Geometry check sheet. Reference: the model listing, model coordinates, mm. A direction names the side the tool comes from. Round coordinates to 2 decimals unless told otherwise and drop trailing zeros. Write each loop counter-clockwise with the first axis right and the second up, starting at its lowest first coordinate (ties: lowest second). Pieces come first, ordered by that corner, then holes. Notation, with made-up numbers: (66, 88) - (88, 88) arc R23 cw to (88, 117) - close; hole circle Ø5 at (-22, 34.5). An arc over 180 degrees is marked (long way). Return JSON: item names as keys, results as strings.
```python
from build123d import *

# Parameters (mm, degrees)
CROQUIS1_R              = 3.1
SALIENTE_EXTRUIR1_DEPTH = 12


with BuildPart() as part:
    # Croquis1 → Saliente-Extruir1 (new body)
    with BuildSketch(Plane.XY):
        Polygon((331.272984938, 614.597621835), (321.632458304, 1225.948656715), (1286.013878227, 1225.948656715), (1286.013878227, 614.597621835), align=None)
        with Locations((1170.33582343, 889.102037351)):
            Circle(CROQUIS1_R, mode=Mode.SUBTRACT)
        with Locations((1220.33582343, 889.102037351)):
            Circle(CROQUIS1_R, mode=Mode.SUBTRACT)
        with Locations((1220.33582343, 953.102037351)):
            Circle(CROQUIS1_R, mode=Mode.SUBTRACT)
        with Locations((1170.33582343, 953.102037351)):
            Circle(CROQUIS1_R, mode=Mode.SUBTRACT)
        with Locations((435.286525189, 859.802037351)):
            Circle(CROQUIS1_R, mode=Mode.SUBTRACT)
        with Locations((370.33582343, 923.276635067)):
            Circle(CROQUIS1_R, mode=Mode.SUBTRACT)
        with Locations((435.286525189, 982.402037351)):
            Circle(CROQUIS1_R, mode=Mode.SUBTRACT)
        with Locations((492.93582343, 923.276635067)):
            Circle(CROQUIS1_R, mode=Mode.SUBTRACT)
        with BuildLine():
            Line((394.578464117, 962.402037351), (468.693182742, 962.402037351))
            ThreePointArc((468.693182742, 962.402037351), (472.93582343, 962.402037351), (472.93582343, 958.159396664))
            Line((472.93582343, 958.159396664), (472.93582343, 884.044678039))
            ThreePointArc((472.93582343, 884.044678039), (472.93582343, 879.802037351), (468.693182742, 879.802037351))
            Line((468.693182742, 879.802037351), (394.578464117, 879.802037351))
            ThreePointArc((394.578464117, 879.802037351), (390.33582343, 879.802037351), (390.33582343, 884.044678039))
            Line((390.33582343, 884.044678039), (390.33582343, 958.159396664))
            ThreePointArc((390.33582343, 958.159396664), (390.33582343, 962.402037351), (394.578464117, 962.402037351))
        make_face(mode=Mode.SUBTRACT)
        with BuildLine():
            Line((742.33582343, 1208.859396664), (742.33582343, 1193.344678039))
            ThreePointArc((742.33582343, 1193.344678039), (742.33582343, 1189.102037351), (738.093182742, 1189.102037351))
            Line((738.093182742, 1189.102037351), (690.578464117, 1189.102037351))
            ThreePointArc((690.578464117, 1189.102037351), (686.33582343, 1189.102037351), (686.33582343, 1193.344678039))
            Line((686.33582343, 1193.344678039), (686.33582343, 1208.859396664))
            ThreePointArc((686.33582343, 1208.859396664), (686.33582343, 1213.102037351), (690.578464117, 1213.102037351))
            Line((690.578464117, 1213.102037351), (738.093182742, 1213.102037351))
            ThreePointArc((738.093182742, 1213.102037351), (742.33582343, 1213.102037351), (742.33582343, 1208.859396664))
        make_face(mode=Mode.SUBTRACT)
        with BuildLine():
            Line((934.33582343, 648.859396664), (934.33582343, 633.344678039))
            ThreePointArc((934.33582343, 633.344678039), (934.33582343, 629.102037351), (930.093182742, 629.102037351))
            Line((930.093182742, 629.102037351), (882.578464117, 629.102037351))
            ThreePointArc((882.578464117, 629.102037351), (878.33582343, 629.102037351), (878.33582343, 633.344678039))
            Line((878.33582343, 633.344678039), (878.33582343, 648.859396664))
            ThreePointArc((878.33582343, 648.859396664), (878.33582343, 653.102037351), (882.578464117, 653.102037351))
            Line((882.578464117, 653.102037351), (930.093182742, 653.102037351))
            ThreePointArc((930.093182742, 653.102037351), (934.33582343, 653.102037351), (934.33582343, 648.859396664))
        make_face(mode=Mode.SUBTRACT)
        with BuildLine():
            Line((690.578464117, 653.102037351), (738.093182742, 653.102037351))
            ThreePointArc((738.093182742, 653.102037351), (742.33582343, 653.102037351), (742.33582343, 648.859396664))
            Line((742.33582343, 648.859396664), (742.33582343, 633.344678039))
            ThreePointArc((742.33582343, 633.344678039), (742.33582343, 629.102037351), (738.093182742, 629.102037351))
            Line((738.093182742, 629.102037351), (690.578464117, 629.102037351))
            ThreePointArc((690.578464117, 629.102037351), (686.33582343, 629.102037351), (686.33582343, 633.344678039))
            Line((686.33582343, 633.344678039), (686.33582343, 648.859396664))
            ThreePointArc((686.33582343, 648.859396664), (686.33582343, 653.102037351), (690.578464117, 653.102037351))
        make_face(mode=Mode.SUBTRACT)
        with BuildLine():
            Line((1220.33582343, 671.102037351), (400.33582343, 671.102037351))
            ThreePointArc((400.33582343, 671.102037351), (393.264755618, 674.03096954), (390.33582343, 681.102037351))
            Line((390.33582343, 681.102037351), (390.33582343, 757.264835053))
            ThreePointArc((390.33582343, 757.264835053), (390.808048943, 760.301529527), (392.180126095, 763.05142308))
            Line((392.180126095, 763.05142308), (443.646345243, 835.588625378))
            ThreePointArc((443.646345243, 835.588625378), (447.212155883, 838.686458556), (451.802042577, 839.802037351))
            Line((451.802042577, 839.802037351), (502.93582343, 839.802037351))
            ThreePointArc((502.93582343, 839.802037351), (510.006891241, 842.73096954), (512.93582343, 849.802037351))
            Line((512.93582343, 849.802037351), (512.93582343, 992.402037351))
            ThreePointArc((512.93582343, 992.402037351), (510.006891241, 999.473105163), (502.93582343, 1002.402037351))
            Line((502.93582343, 1002.402037351), (451.802042577, 1002.402037351))
            ThreePointArc((451.802042577, 1002.402037351), (447.212155883, 1003.517616147), (443.646345243, 1006.615449325))
            Line((443.646345243, 1006.615449325), (392.180126095, 1079.152651623))
            ThreePointArc((392.180126095, 1079.152651623), (390.808048943, 1081.902545176), (390.33582343, 1084.93923965))
            Line((390.33582343, 1084.93923965), (390.33582343, 1161.102037351))
            ThreePointArc((390.33582343, 1161.102037351), (393.264755618, 1168.173105163), (400.33582343, 1171.102037351))
            Line((400.33582343, 1171.102037351), (1220.33582343, 1171.102037351))
            ThreePointArc((1220.33582343, 1171.102037351), (1227.406891241, 1168.173105163), (1230.33582343, 1161.102037351))
            Line((1230.33582343, 1161.102037351), (1230.33582343, 1068.903333434))
            ThreePointArc((1230.33582343, 1068.903333434), (1230.177434198, 1067.130567942), (1229.707283932, 1065.413959843))
            Line((1229.707283932, 1065.413959843), (1197.759992837, 979.61266376))
            ThreePointArc((1197.759992837, 979.61266376), (1194.094067546, 974.889433139), (1188.388532335, 973.102037351))
            Line((1188.388532335, 973.102037351), (1160.33582343, 973.102037351))
            ThreePointArc((1160.33582343, 973.102037351), (1153.264755618, 970.173105163), (1150.33582343, 963.102037351))
            Line((1150.33582343, 963.102037351), (1150.33582343, 943.102037351))
            ThreePointArc((1150.33582343, 943.102037351), (1153.264755618, 936.03096954), (1160.33582343, 933.102037351))
            Line((1160.33582343, 933.102037351), (1220.33582343, 933.102037351))
            ThreePointArc((1220.33582343, 933.102037351), (1227.406891241, 930.173105163), (1230.33582343, 923.102037351))
            Line((1230.33582343, 923.102037351), (1230.33582343, 919.102037351))
            ThreePointArc((1230.33582343, 919.102037351), (1227.406891241, 912.03096954), (1220.33582343, 909.102037351))
            Line((1220.33582343, 909.102037351), (1160.33582343, 909.102037351))
            ThreePointArc((1160.33582343, 909.102037351), (1153.264755618, 906.173105163), (1150.33582343, 899.102037351))
            Line((1150.33582343, 899.102037351), (1150.33582343, 879.102037351))
            ThreePointArc((1150.33582343, 879.102037351), (1153.264755618, 872.03096954), (1160.33582343, 869.102037351))
            Line((1160.33582343, 869.102037351), (1188.388532335, 869.102037351))
            ThreePointArc((1188.388532335, 869.102037351), (1194.094067546, 867.314641564), (1197.759992837, 862.591410943))
            Line((1197.759992837, 862.591410943), (1229.707283932, 776.79011486))
            ThreePointArc((1229.707283932, 776.79011486), (1230.177434198, 775.073506761), (1230.33582343, 773.300741269))
            Line((1230.33582343, 773.300741269), (1230.33582343, 681.102037351))
            ThreePointArc((1230.33582343, 681.102037351), (1227.406891241, 674.03096954), (1220.33582343, 671.102037351))
        make_face(mode=Mode.SUBTRACT)
        with BuildLine():
            Line((786.578464117, 653.102037351), (834.093182742, 653.102037351))
            ThreePointArc((834.093182742, 653.102037351), (838.33582343, 653.102037351), (838.33582343, 648.859396664))
            Line((838.33582343, 648.859396664), (838.33582343, 635.344678039))
            ThreePointArc((838.33582343, 635.344678039), (838.33582343, 631.102037351), (834.093182742, 631.102037351))
            Line((834.093182742, 631.102037351), (786.578464117, 631.102037351))
            ThreePointArc((786.578464117, 631.102037351), (782.33582343, 631.102037351), (782.33582343, 635.344678039))
            Line((782.33582343, 635.344678039), (782.33582343, 648.859396664))
            ThreePointArc((782.33582343, 648.859396664), (782.33582343, 653.102037351), (786.578464117, 653.102037351))
        make_face(mode=Mode.SUBTRACT)
        with BuildLine():
            Line((934.33582343, 1208.859396664), (934.33582343, 1193.344678039))
            ThreePointArc((934.33582343, 1193.344678039), (934.33582343, 1189.102037351), (930.093182742, 1189.102037351))
            Line((930.093182742, 1189.102037351), (882.578464117, 1189.102037351))
            ThreePointArc((882.578464117, 1189.102037351), (878.33582343, 1189.102037351), (878.33582343, 1193.344678039))
            Line((878.33582343, 1193.344678039), (878.33582343, 1208.859396664))
            ThreePointArc((878.33582343, 1208.859396664), (878.33582343, 1213.102037351), (882.578464117, 1213.102037351))
            Line((882.578464117, 1213.102037351), (930.093182742, 1213.102037351))
            ThreePointArc((930.093182742, 1213.102037351), (934.33582343, 1213.102037351), (934.33582343, 1208.859396664))
        make_face(mode=Mode.SUBTRACT)
        with BuildLine():
            Line((838.33582343, 1206.859396664), (838.33582343, 1193.344678039))
            ThreePointArc((838.33582343, 1193.344678039), (838.33582343, 1189.102037351), (834.093182742, 1189.102037351))
            Line((834.093182742, 1189.102037351), (786.578464117, 1189.102037351))
            ThreePointArc((786.578464117, 1189.102037351), (782.33582343, 1189.102037351), (782.33582343, 1193.344678039))
            Line((782.33582343, 1193.344678039), (782.33582343, 1206.859396664))
            ThreePointArc((782.33582343, 1206.859396664), (782.33582343, 1211.102037351), (786.578464117, 1211.102037351))
            Line((786.578464117, 1211.102037351), (834.093182742, 1211.102037351))
            ThreePointArc((834.093182742, 1211.102037351), (838.33582343, 1211.102037351), (838.33582343, 1206.859396664))
        make_face(mode=Mode.SUBTRACT)
    extrude(amount=SALIENTE_EXTRUIR1_DEPTH)


solid = part.part
```
(1) Material ranges on line 1 along Y through (x, z) = (472, 5.5); line 2 along Y through (x, z) = (724, 5.25); line 3 along Y through (x, z) = (843, 1.5), recorded low to high. Write a range as [from, to].
Response values:
{"line 1": "y = [614.6, 671.1], [839.8, 879.17], [963.04, 1002.4], [1171.1, 1225.95]", "line 2": "y = [614.6, 629.1], [653.1, 671.1], [1171.1, 1189.1], [1213.1, 1225.95]", "line 3": "y = [614.6, 671.1], [1171.1, 1225.95]"}
(2) Section check A-A, the plane y = 722. Enter the section's corners in (x, z).
Response values:
{"outline": "(329.58, 0) - (390.34, 0) - (390.34, 12) - (329.58, 12) - close; (1230.34, 0) - (1286.01, 0) - (1286.01, 12) - (1230.34, 12) - close"}
(3) Gauge pin test, flat ends, axial feed: pin 1 (5 mm diameter, centred on x = 1170.34, y = 889.1, fed in from +Z); pin 2 (2 mm diameter, centred on y = 921, z = 6, fed in from -X); pin 3 (6 mm diameter, centred on y = 1111, z = 3, fed in from -X); pin 4 (3 mm diameter, centred on y = 692.5, z = 7, fed in from -X). Record the tip position at first contact, or that the pin passes through.
Response values:
{"pin 1": "passes through", "pin 2": "stops at x = 326.43", "pin 3": "stops at x = 323.4", "pin 4": "stops at x = 330.02"}
(4) Release check for a two-part mould opening along Y. For faces 3 (the face through (1213.51, 820.29, 5.92)), 4 (the face through (842, 1193, 12)) record: pulls with the +Y half, pulls with the -Y half, needs draft (parallel to the pull), parting line crosses it, or undercut.
Response values:
{"face 3": "undercut", "face 4": "needs draft"}
(5) Section check B-B, the plane x = 628.5. Enter the section's corners in (y, z).
Response values:
{"outline": "(614.6, 0) - (671.1, 0) - (671.1, 12) - (614.6, 12) - close; (1171.1, 0) - (1225.95, 0) - (1225.95, 12) - (1171.1, 12) - close"}
(6) Access from +Z, -Z, +X, -X, +Y, -Y to the whole of each face (thin tool, end or side, straight path). Record for faces 1 (the face through (1213.957, 1023.114, 5.916)), 2 (the face through (842, 1193, 0)).
Response values:
{"face 1": "+Z, -Z", "face 2": "-Z, +X, -X, +Y, -Y"}
(7) Section check C-C, the plane z = 2.5. Give the number of separate pieces and of enclosed holes in the cut face, plus the area to 3 significant figures.
Response values:
{"separate pieces": "1", "enclosed holes": "16", "area": "186,000 mm^2"}
